Part model, mm, in its own coordinate system. Face numbers are marked on the shaded views. A direction names the side the tool comes from. Coordinates: 2 decimals unless noted, no trailing zeros. Loops run counter-clockwise (first coordinate to the right, second up) from the corner with the lowest first, then second, coordinate; pieces in that order, holes last. Notation, with made-up numbers: (51, 57) - (88, 57) arc R18 cw to (88, 86) - close; hole circle Ø1 at (77.25, 18.5). An arc over 180 degrees is marked (long way). Use a Markdown table: item, result. Add a question column.
1) Pull direction Z, two halves, no side cores. Call the marked faces 1, 2 and 3: +Z half, -Z half, draft (parallel to the pull), parting line (faces both ways), or undercut.
2) Band-saw the part on C-C (y = 15.75). Give the number of separate pieces and of enclosed holes in the cut face, plus the area to 3 significant figures.
3) Probe probe 1 along X at (y, z) = (8.5, 0); probe 2 along X at (y, z) = (10, 7.5); probe 3 along Z at (x, y) = (-0.5, 14.75). List the from-to ranges inside material, lowest first. Write a range as [from, to].
4) Drop flat-ended pins along their axis: P1, Ø4.5, axis at x = -17.88, z = 20.23, coming from the -Y side; P2, Ø6.5, axis at x = -8.58, z = -25.6, coming from the -Y side; P3, Ø3, axis at y = 7, z = -7.5, coming from the -X side; P4, Ø8, axis at y = 10, z = -19, coming from the +X side. Give the stop position or say it passes through.
5) Tool access for the marked faces 4 and 5: list every direction of +Z, -Z, +X, -X, +Y, -Y with a clear straight run to the whole face (end or side of a thin tool).
6) Band-saw the part on A-A (z = -12.5). Give the cut face in (x, y) (3 decimals), plus the area to 3 significant figures.
Autodesk Inventor part; units mm, degrees
ref_plane "YZ Plane" through (0, 0, 0) normal (1, 0, 0) x (0, 1, 0)
ref_plane "XZ Plane" through (0, 0, 0) normal (0, 1, 0) x (-1, 0, 0)
ref_plane "XY Plane" through (0, 0, 0) normal (0, 0, 1) x (1, 0, 0)
sketch "Sketch1" plane through (0, 0, 0) normal (0, 1, 0) x (-1, 0, 0)
  circle A0 centre (0, 0) radius 22.5
  circle A1 centre (0, 0) radius 37.5
  dimension "d0" = 45
  dimension "d1" = 75
extrude "Extrusion1" add sketch "Sketch1" along normal blind 2
sketch "Sketch2" plane through (0, 2, 0) normal (0, 1, 0) x (1, 0, 0)
  circle A0 centre (0, 0) radius 37.5
  circle A1 centre (0, 0) radius 22.5
  circle A2 centre (0, 0) radius 32.4
  dimension "d4" = 64.8
extrude "Extrusion2" add sketch "Sketch2" along normal blind 15.875 contours A2
feature "FaceDraft1" [suppressed]
sketch "Sketch3" plane through (0, 17.875, 0) normal (0, 1, 0) x (1, 0, 0)
  circle A0 centre (26.4608, -5.3692) radius 2.875
  circle A1 centre (17.8802, 20.2311) radius 2.875
  circle A2 centre (-8.5805, 25.6003) radius 2.875
  circle A3 centre (-26.4608, 5.3692) radius 2.875
  circle A4 centre (-17.8802, -20.2311) radius 2.875
  circle A5 centre (8.5805, -25.6003) radius 2.875
  point P0 (0, 0)
extrude "Extrusion3" cut sketch "Sketch3" against normal through all
sketch "Sketch4" plane through (0, 0, 0) normal (0, -1, 0) x (1, 0, 0)
  circle A0 centre (26.4608, 5.3692) radius 2.875
  line L0 (30.7783, 3.7285) -> (27.1986, 0.8097)
  line L1 (27.1986, 0.8097) -> (22.8811, 2.4504)
  line L2 (22.8811, 2.4504) -> (22.1432, 7.0099)
  line L3 (22.1432, 7.0099) -> (25.7229, 9.9287)
  line L4 (25.7229, 9.9287) -> (30.0404, 8.2879)
  line L5 (30.0404, 8.2879) -> (30.7783, 3.7285)
  point P0 (0, 0)
  dimension "d10" = 8
extrude "Extrusion4" cut sketch "Sketch4" against normal blind 5 contours A0 | L0 L1 L2 L3 L4 L5
pattern_circular "Circular Pattern1" count 6 over 360 about axis through (0, 2, 0) along (0, 1, 0) of "Extrusion4"
properties part number "j1FlangeV2"
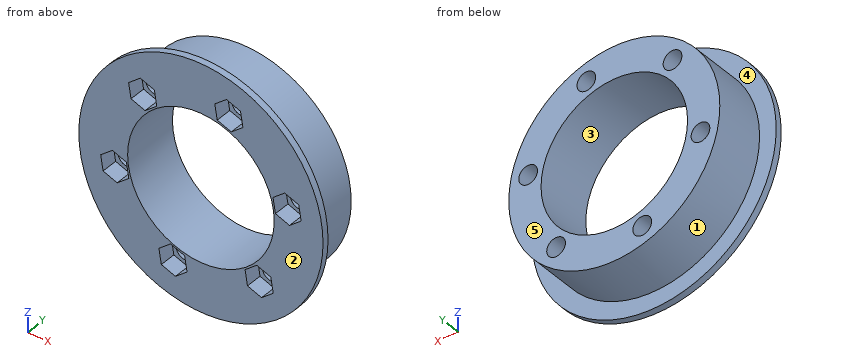
Answer block:
| question | item | result |
|---|---|---|
| 1 | face 1 | parting line |
| 1 | face 2 | draft |
| 1 | face 3 | undercut |
| 2 | separate pieces | 1 |
| 2 | enclosed holes | 7 |
| 2 | area | 1,550 mm2 |
| 3 | probe 1 | [-32.4, -22.5], [22.5, 32.4] |
| 3 | probe 2 | [-31.52, -21.21], [21.21, 24.53], [28.39, 31.52] |
| 3 | probe 3 | [-32.4, -22.49], [22.49, 32.4] |
| 4 | P1 | through |
| 4 | P2 | y = 5 |
| 4 | P3 | x = -31.84 |
| 4 | P4 | x = 28.72 |
| 5 | face 4 | +Y |
| 5 | face 5 | +Z, -Z, +X, -X, +Y |
| 6 | outline | (-35.355, 0) - (-18.708, 0) - (-18.708, 17.875) - (-29.892, 17.875) - (-29.892, 2) - (-35.355, 2) - close; (18.708, 0) - (35.355, 0) - (35.355, 2) - (29.892, 2) - (29.892, 17.875) - (18.708, 17.875) - close |
| 6 | area | 422 mm2 |
